The listing builds one solid part. Answer for the finished solid, in the listing's coordinates (mm). A direction names the side the tool comes from. Give positions to 0.01 mm unless a question says otherwise; leave off trailing zeros. Order: outer loops, then holes, each group sorted by start corner. A loop starts at its lowest first (then second) coordinate and runs counter-clockwise, first axis right, second up. Notation, with made-up numbers: (-9.75, 52.5) - (32.25, 52.5) arc R17 ccw to (32.25, 83.5) - close; hole circle Ø4 at (-28.75, 68.5). An arc over 180 degrees is marked (long way). Write each question's results on one line, items separated by ' | '. Start each with the question number.
1. Find the intervals of material crossed by L1, parallel to Y at x = -23.5, z = 17.4; L2, parallel to Z at x = 15, y = -0.75; L3, parallel to X at y = -0.75, z = -16, in increasing order.
2. Determine the mould class of faces 1 (the face through (26.359, 2.797, 18.944)), 2 (the face through (-26.297, 2.859, -18.944)), 3 (the face through (21.75, 0.08, -18.94)), 4 (the face through (31.316, 10.433, -21.902)) for opening direction X: released by +X, released by -X, zero draft, split by the parting line, or undercut.
3. Flat-ended cylindrical pins translate along their axes: pin 1 (2.5 mm diameter, centred on x = 19, y = 2, fed in from -Z); pin 2 (1.9 mm diameter, centred on x = -22.5, y = 1, fed in from +Z); pin 3 (4 mm diameter, centred on x = -6, z = -15, fed in from +Y); pin 4 (4 mm diameter, centred on y = 12, z = -18.5, fed in from +X). Find the tip coordinate at first contact, or state that the pin passes through.
4. Section C-C (z = -10) is taken. Give the vertices of the cut face in (x, y).
5. Section D-D (x = -3) is taken. Give the vertices of the cut face in (y, z), and give its area (3 significant figures).
6. Section B-B (z = -18) is taken. State how many separate pieces and enclosed holes the cut face has, and give its area (3 significant figures).
7. Which of the six approach directions +Z, -Z, +X, -X, +Y, -Y give full straight-line access (tool end or side, diameter ignored) to faces 5 (the face through (-4.9, 0.06, 14.14)), 6 (the face through (17, 0, 15)), 7 (the face through (29.744, 14.506, -23.458)), 8 (the face through (28, 12, -29))?
8. Section A-A (x = -18) is taken. Give the vertices of the cut face in (y, z), and give its area (3 significant figures).
from build123d import *

# Parameters (mm, degrees)
SALIENTE_EXTRUIR1_DEPTH = 4
CROQUIS3_R              = 1.75
CORTAR_EXTRUIR1_DEPTH   = 54.742441329
REDONDEO8_R             = 4
REDONDEO9_R             = 3
SALIENTE_EXTRUIR3_START = -8
CROQUIS5_R              = 1.75
SALIENTE_EXTRUIR3_DEPTH = 8
CROQUIS4_R              = 4
CROQUIS4_R_2            = 1.75
SALIENTE_EXTRUIR2_DEPTH = 6
CROQUIS6_R              = 3.1
CORTAR_EXTRUIR2_DEPTH   = 3.2


with BuildPart() as part:
    # Croquis2 → Saliente-Extruir1 (new, symmetric)
    with BuildSketch(Plane(origin=(0, 0, 0), x_dir=(1, 0, 0), z_dir=(0, 1, 0))):
        Polygon((27.5, -23), (27.5, -15), (4, -15), (4, 15), (27.5, 15), (27.5, 23), (-27.5, 23), (-27.5, 15), (-4, 15), (-4, -15), (-27.5, -15), (-27.5, -23), align=None)
    extrude(amount=SALIENTE_EXTRUIR1_DEPTH, both=True)

    # Croquis3 → Cortar-Extruir1 (cut, through all)
    with BuildSketch(Plane.XY.offset(23)):
        with Locations((23.5, 0)):
            Circle(CROQUIS3_R)
        with Locations((-23.5, 0)):
            Circle(CROQUIS3_R)
    extrude(amount=-CORTAR_EXTRUIR1_DEPTH, mode=Mode.SUBTRACT)

    # Redondeo8
    redondeo8_edges = [part.edges().sort_by_distance(p)[0] for p in [
        (27.5, -4, -19),
        (27.5, 4, -19),
        (27.5, -4, 19),
        (27.5, 4, 19),
        (-27.5, -4, -19),
        (-27.5, 4, -19),
        (-27.5, -4, 19),
        (-27.5, 4, 19),
    ]]
    fillet(redondeo8_edges, radius=REDONDEO8_R - 0.0001)  # a hair under: the kernel refuses the full size

    # Redondeo9
    redondeo9_edges = [part.edges().sort_by_distance(p)[0] for p in [
        (4, 0, -15),
        (4, 0, 15),
        (-4, 0, 15),
        (-4, 0, -15),
    ]]
    fillet(redondeo9_edges, radius=REDONDEO9_R)

    # Croquis5 → Saliente-Extruir3 (add)
    with BuildSketch(Plane(origin=(0, 0, -23), x_dir=(-1, 0, 0), z_dir=(0, 0, -1)).offset(SALIENTE_EXTRUIR3_START)):
        with BuildLine():
            Line((-26.103713296, 12.509763717), (-20.035898385, 2))
            ThreePointArc((-20.035898385, 2), (-21.5, -3.464101615), (-26.964101615, -2))
            Line((-26.964101615, -2), (-33.031916526, 8.509763717))
            ThreePointArc((-33.031916526, 8.509763717), (-31.567814911, 13.973865332), (-26.103713296, 12.509763717))
        make_face()
        with Locations(Location((-23.5, 0, 0), (0, 0, 180))):
            Circle(CROQUIS5_R, mode=Mode.SUBTRACT)
        with Locations((-29.567814911, 10.509763717)):
            Circle(CROQUIS5_R, mode=Mode.SUBTRACT)
    extrude(amount=SALIENTE_EXTRUIR3_DEPTH)

    # Croquis4 → Saliente-Extruir2 (add)
    with BuildSketch(Plane.XY.offset(-23)):
        with Locations(Location((29.567814911, 10.509763717, 0), (0, 0, 150))):
            Circle(CROQUIS4_R)
        with Locations(Location((29.567814911, 10.509763717, 0), (0, 0, 180))):
            Circle(CROQUIS4_R_2, mode=Mode.SUBTRACT)
    extrude(amount=-SALIENTE_EXTRUIR2_DEPTH)

    # Croquis6 → Cortar-Extruir2 (cut)
    with BuildSketch(Plane.XY.offset(23)):
        with Locations((-23.5, 0)):
            Circle(CROQUIS6_R)
    extrude(amount=-CORTAR_EXTRUIR2_DEPTH, mode=Mode.SUBTRACT)


solid = part.part
Reported:
1) L1: -4 to -1.75, 1.75 to 4 | L2: -23 to -15, 15 to 23 | L3: -27.43 to -25.08, -21.92 to 21.92, 25.08 to 27.69
2) face 1: released by +X | face 2: released by -X | face 3: undercut | face 4: undercut
3) pin 1: z = -23 | pin 2: z = 19.8 | pin 3: y = 4 | pin 4: x = 33.57
4) outline: (-4, -4) - (4, -4) - (4, 4) - (-4, 4) - close
5) outline: (-4, -23) - (4, -23) - (4, 23) - (-4, 23) - close | area: 368 mm²
6) separate pieces: 1 | enclosed holes: 3 | area: 494 mm²
7) face 5: -X, +Y, -Y | face 6: +X, +Y, -Y | face 7: -Z | face 8: -Z, +X, -X, +Y, -Y
8) outline: (-4, -23) - (4, -23) - (4, -15) - (-4, -15) - close; (-4, 15) - (4, 15) - (4, 23) - (-4, 23) - close | area: 128 mm²
